```python
from build123d import *

# Parameters (mm, degrees)
F1_DEPTH = 990.6
F2_R     = 4.7625
F3_DEPTH = 38.101


with BuildPart() as f1:
    # F0 (on Front) → F1 (new body)
    with BuildSketch(Plane.XZ):
        Polygon((38.1, 0), (0, 0), (0, -3.175), (34.925, -3.175), (34.925, -38.1), (38.1, -38.1), align=None)
    extrude(amount=F1_DEPTH)

    # F2 (on face) → F3 (cut, through all)
    with BuildSketch(Plane.XY):
        with Locations((12.7, -927.1)):
            Circle(F2_R)
        with Locations((12.7, -787.4)):
            Circle(F2_R)
        with Locations((12.7, -203.2)):
            Circle(F2_R)
        with Locations((12.7, -63.5)):
            Circle(F2_R)
    extrude(amount=-F3_DEPTH, mode=Mode.SUBTRACT)


solid = f1.part
```
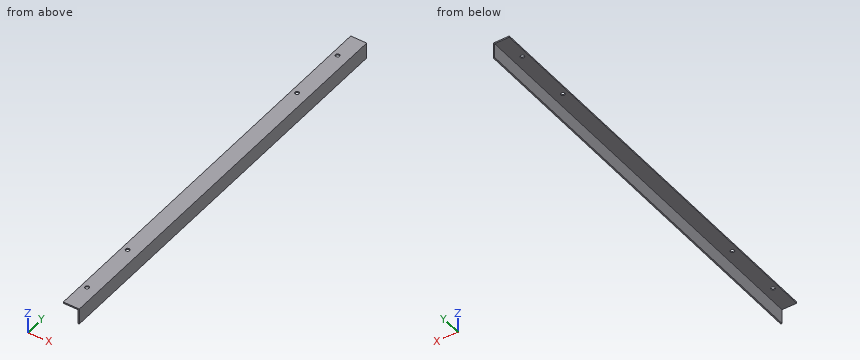
Input: part model. Units: mm. Frame: model coordinates. Give positions to 0.01 mm unless a question says otherwise; leave off trailing zeros. Order: outer loops, then holes, each group sorted by start corner. A loop starts at its lowest first (then second) coordinate and runs counter-clockwise, first axis right, second up. Notation, with made-up numbers: (-24, 8) - (10, 8) arc R23 cw to (10, 31) - close; hole circle Ø3 at (-35.75, 5.5). An arc over 180 degrees is marked (long way). Use a Markdown table: item, result.
(1) Section query A-A (y = -359). Output: boundary loops of the cut face in (x, z) (3 decimals), then the cut area to 3 significant figures.
Computed values:
| item | result |
|---|---|
| outline | (0, -3.175) - (34.925, -3.175) - (34.925, -38.1) - (38.1, -38.1) - (38.1, 0) - (0, 0) - close |
| area | 232 mm2 |
(2) Section query B-B (z = -15). Output: boundary loops of the cut face in (x, y) (3 decimals).
Computed values:
| item | result |
|---|---|
| outline | (34.925, -990.6) - (38.1, -990.6) - (38.1, 0) - (34.925, 0) - close |
(3) Line query: line 1 (Y direction, x = 12, z = -1); line 2 (Y direction, x = 12.7, z = -1.95); line 3 (X direction, y = -927.1, z = -1.75). Output: solid intervals per line, ascending. Write a range as from..to.
Computed values:
| item | result |
|---|---|
| line 1 | y = -990.6..-931.81, -922.39..-792.11, -782.69..-207.91, -198.49..-68.21, -58.79..0 |
| line 2 | y = -990.6..-931.86, -922.34..-792.16, -782.64..-207.96, -198.44..-68.26, -58.74..0 |
| line 3 | x = 0..7.94, 17.46..38.1 |
(4) Pin query (flat end, axial travel): pin 1 (10 mm diameter, centred on y = -706.5, z = -12, fed in from -X) (3 decimals); pin 2 (5.5 mm diameter, centred on x = 12.7, y = -203.2, fed in from +Z). Return the tip coordinate at first contact, or that it passes through.
Computed values:
| item | result |
|---|---|
| pin 1 | stops at x = 34.925 |
| pin 2 | passes through |
